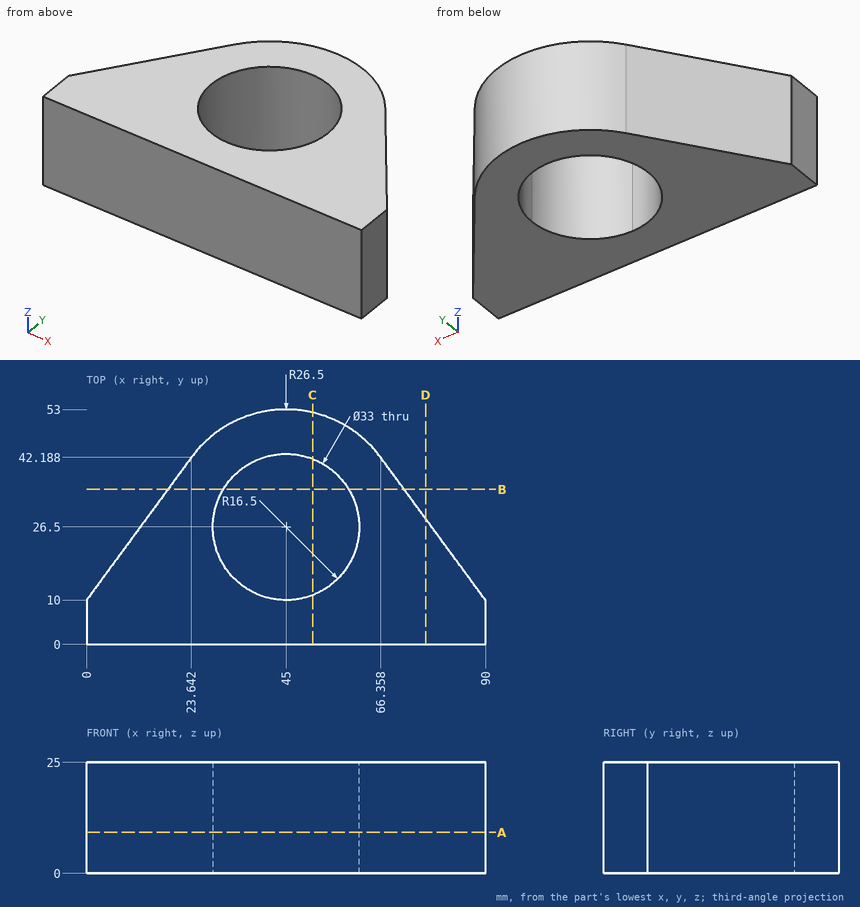
The drawing under review shows one solid part. Ordinate dimensions are in mm from its lowest x, y, z. Round coordinates to 2 decimals unless told otherwise and drop trailing zeros. Loops run counter-clockwise (first coordinate to the right, second up) from the corner with the lowest first, then second, coordinate; pieces in that order, holes last. Notation, with made-up numbers: (-2.5, 81.5) - (40.5, 81.5) arc R16 ccw to (40.5, 104.5) - close; hole circle Ø10 at (-8, 8.5). An arc over 180 degrees is marked (long way). Use a Markdown table: item, result. Add a question column.
Q1. For probe 1 along Y at (x, z) = (45, 9); probe 2 along X at (y, z) = (27.5, 5.5) (1 decimal); probe 3 along X at (y, z) = (37, 18), list the stretches that pass through material, from the lowest coordinate up.
Q2. Add section C-C (x = 51). State the section outline as (y, z) points, plus the area to 3 significant figures.
Q3. Add section B-B (y = 35). State the section outline as (x, z) points.
Q4. Add section A-A (z = 9.25). State the section outline as (x, y) points.
Q5. Insertion check: pin 1 Ø5 at (y, z) = (20.5, 17) entering from -X (1 decimal); pin 2 Ø6 at (x, z) = (46, 16) entering from +Y; pin 3 Ø10 at (y, z) = (35, 8) entering from +X. Each pin has a flat end and moves straight along its axis. Give the tip position at first contact, or say it passes through.
Q6. Add section D-D (x = 76.5). State the section outline as (y, z) points.
Worked answers:
| question | item | result |
|---|---|---|
| 1 | probe 1 | 0 to 10, 43 to 53 |
| 1 | probe 2 | 12.9 to 28.5, 61.5 to 77.1 |
| 1 | probe 3 | 19.83 to 32.27, 57.73 to 70.17 |
| 2 | outline | (0, 0) - (11.13, 0) - (11.13, 25) - (0, 25) - close; (41.87, 0) - (52.31, 0) - (52.31, 25) - (41.87, 25) - close |
| 2 | area | 539 mm² |
| 3 | outline | (18.36, 0) - (30.86, 0) - (30.86, 25) - (18.36, 25) - close; (59.14, 0) - (71.64, 0) - (71.64, 25) - (59.14, 25) - close |
| 4 | outline | (0, 0) - (90, 0) - (90, 10) - (66.36, 42.19) arc R26.5 ccw to (23.64, 42.19) - (0, 10) - close; hole circle Ø33 at (45, 26.5) |
| 5 | pin 1 | x = 5.9 |
| 5 | pin 2 | y = 53 |
| 5 | pin 3 | x = 75.31 |
| 6 | outline | (0, 0) - (28.38, 0) - (28.38, 25) - (0, 25) - close |
